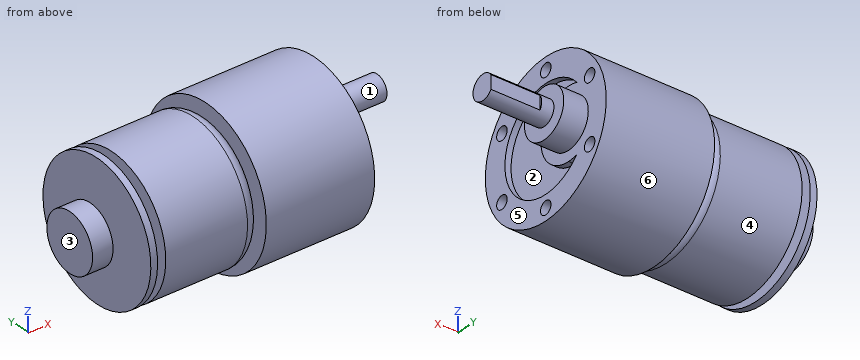
from build123d import *

# Parameters (mm, degrees)
CROQUIS_MOTOR_BASE_R      = 16.5
SALIENTE_EXTRUIR1_DEPTH   = 23
REDONDEO1_R               = 3
CROQUIS_REDUCTOR_BASE_R   = 18.5
SALIENTE_EXTRUIR2_DEPTH   = 26.5
CROQUIS_MOTOR_SHAFT_R     = 6
SALIENTE_EXTRUIR3_DEPTH   = 6
CORTAR_EXTRUIR1_DEPTH     = 1.5
CROQUIS_SHAFT_R           = 3
SALIENTE_EXTRUIR4_DEPTH   = 15
CORTAR_EXTRUIR2_START     = -12
CORTAR_EXTRUIR2_DEPTH     = 12
CROQUIS_MOUNT_AND_CLOSE_R = 1.6
CORTAR_EXTRUIR3_DEPTH     = 3
CROQUIS_MOTOR_SHAFT_OUT_R = 4
SALIENTE_EXTRUIR5_DEPTH   = 2
SALIENTE_EXTRUIR6_START   = 1.65
CROQUIS_ELECTRONICS_R     = 16.5
SALIENTE_EXTRUIR6_DEPTH   = 1.65
CROQUIS_MOTOR_AXIS_R      = 1
SALIENTE_EXTRUIR7_DEPTH   = 1.65
CROQUIS_ENCODER_R         = 7
SALIENTE_EXTRUIR8_DEPTH   = 5


with BuildPart() as part:
    # Croquis motor base → Saliente-Extruir1 (new body)
    with BuildSketch(Plane(origin=(0, 0, 0), x_dir=(0, 0, -1), z_dir=(1, 0, 0))):
        Circle(CROQUIS_MOTOR_BASE_R)
    extrude(amount=SALIENTE_EXTRUIR1_DEPTH)

    # Redondeo1
    redondeo1_edges = [part.edges().sort_by_distance(p)[0] for p in [
        (23, 0, 16.5),
    ]]
    fillet(redondeo1_edges, radius=REDONDEO1_R)

    # Croquis reductor base → Saliente-Extruir2 (add)
    with BuildSketch(Plane(origin=(23, 0, 0), x_dir=(0, 0, -1), z_dir=(1, 0, 0))):
        Circle(CROQUIS_REDUCTOR_BASE_R)
    extrude(amount=SALIENTE_EXTRUIR2_DEPTH)

    # Croquis motor shaft → Saliente-Extruir3 (add)
    with BuildSketch(Plane(origin=(49.5, 0, 0), x_dir=(0, 0, -1), z_dir=(1, 0, 0))):
        with Locations((0, 7)):
            Circle(CROQUIS_MOTOR_SHAFT_R)
    extrude(amount=SALIENTE_EXTRUIR3_DEPTH)

    # Croquis motor shaft_3 → Cortar-Extruir1 (cut)
    with BuildSketch(Plane(origin=(49.5, 0, 0), x_dir=(0, 0, -1), z_dir=(1, 0, 0))):
        with BuildLine():
            ThreePointArc((8.124038405, 9.5), (8.405484116, 8.264055687), (8.5, 7))
            ThreePointArc((8.5, 7), (-1.264055687, -1.405484116), (-8.124038405, 9.5))
            ThreePointArc((-8.124038405, 9.5), (0, -12.5), (8.124038405, 9.5))
        make_face()
    extrude(amount=-CORTAR_EXTRUIR1_DEPTH, mode=Mode.SUBTRACT)

    # Croquis shaft → Saliente-Extruir4 (add)
    with BuildSketch(Plane(origin=(55.5, 0, 0), x_dir=(0, 0, -1), z_dir=(1, 0, 0))):
        with Locations((0, 7)):
            Circle(CROQUIS_SHAFT_R)
    extrude(amount=SALIENTE_EXTRUIR4_DEPTH)

    # Croquis shaft lock → Cortar-Extruir2 (cut)
    with BuildSketch(Plane(origin=(70.5, 0, 0), x_dir=(0, 0, -1), z_dir=(1, 0, 0)).offset(CORTAR_EXTRUIR2_START)):
        with BuildLine():
            Line((-1.658312395, 9.5), (1.658312395, 9.5))
            ThreePointArc((1.658312395, 9.5), (0, 10), (-1.658312395, 9.5))
        make_face()
    extrude(amount=CORTAR_EXTRUIR2_DEPTH, mode=Mode.SUBTRACT)

    # Croquis mount and close → Cortar-Extruir3 (cut)
    with BuildSketch(Plane(origin=(49.5, 0, 0), x_dir=(0, 0, -1), z_dir=(1, 0, 0))):
        with Locations((-15.5, 0)):
            Circle(CROQUIS_MOUNT_AND_CLOSE_R)
        with Locations((-7.75, 13.423393759)):
            Circle(CROQUIS_MOUNT_AND_CLOSE_R)
        with Locations((7.75, 13.423393759)):
            Circle(CROQUIS_MOUNT_AND_CLOSE_R)
        with Locations((15.5, 0)):
            Circle(CROQUIS_MOUNT_AND_CLOSE_R)
        with Locations((7.75, -13.423393759)):
            Circle(CROQUIS_MOUNT_AND_CLOSE_R)
        with Locations((-7.75, -13.423393759)):
            Circle(CROQUIS_MOUNT_AND_CLOSE_R)
    extrude(amount=-CORTAR_EXTRUIR3_DEPTH, mode=Mode.SUBTRACT)

    # Croquis motor shaft out → Saliente-Extruir5 (add)
    with BuildSketch(Plane.ZY):
        Circle(CROQUIS_MOTOR_SHAFT_OUT_R)
    extrude(amount=SALIENTE_EXTRUIR5_DEPTH)

    # Croquis electronics → Saliente-Extruir6 (add)
    with BuildSketch(Plane.ZY.offset(2).offset(SALIENTE_EXTRUIR6_START)):
        with Locations(Location((0, 0, 0), (0, 0, 180))):
            Circle(CROQUIS_ELECTRONICS_R)
    extrude(amount=-SALIENTE_EXTRUIR6_DEPTH)

    # Croquis motor axis → Saliente-Extruir7 (add)
    with BuildSketch(Plane.ZY.offset(3.65)):
        Circle(CROQUIS_MOTOR_AXIS_R)
    extrude(amount=SALIENTE_EXTRUIR7_DEPTH)

    # Croquis encoder → Saliente-Extruir8 (add)
    with BuildSketch(Plane.ZY.offset(5.3)):
        Circle(CROQUIS_ENCODER_R)
    extrude(amount=SALIENTE_EXTRUIR8_DEPTH)


solid = part.part
Input: part model. Units: mm. Frame: model coordinates. Face numbers are marked on the shaded views. A direction names the side the tool comes from. Give positions to 0.01 mm unless a question says otherwise; leave off trailing zeros. Write each loop counter-clockwise with the first axis right and the second up, starting at its lowest first coordinate (ties: lowest second). Pieces come first, ordered by that corner, then holes. Notation, with made-up numbers: M 29,-13.75 L 81,-13.75 A24 cw 81,5.25 Z; hole C -38.5,67 d11. An arc over 180 degrees is marked long. Write item = value, one per line. Start each with the question number.
1) First-contact query: pin 1 Ø2 at (y, z) = (-1.5, -2) entering from +X; pin 2 Ø2.5 at (y, z) = (13.42, 7.75) entering from +X; pin 3 Ø8 at (x, z) = (25.5, -6.5) entering from +Y. Flat tips, straight axial feed; report the tip coordinate or a pass-through.
2) Draft query along Y for the marked faces 1, 2 and 3. Return one class per face: +Y half, -Y half, draft (parallel to the pull), parting line (faces both ways), or undercut.
3) Material intervals for line 1 along X through (y, z) = (-7, -8.5); line 2 along X through (y, z) = (-5, 11.5); line 3 along Y through (x, z) = (48.1, -7.75), sorted ascending. Write a range as [from, to].
4) Reachability of the marked faces 4, 5 and 6 from +Z, -Z, +X, -X, +Y, -Y: full face, straight path, thin tool, end or side. Return the list, or none.
5) Cut plane A-A on z = -15.5. Count the separate pieces of the cut face and the enclosed holes in it, then the cut area to 3 significant figures.
6) Cut plane B-B on x = 8. Return the cut outline in (y, z), then the cut area to 3 significant figures.
Solved:
q1.pin_1 = 49.5
q1.pin_2 = 46.5
q1.pin_3 = 18.33
q2.face_1 = parting line
q2.face_2 = undercut
q2.face_3 = draft
q3.line_1 = [-3.65, -2], [0, 48]
q3.line_2 = [-3.65, -2], [0, 49.5]
q3.line_3 = [-16.8, -15.02], [-11.82, -9.81], [3.51, 11.82], [15.02, 16.8]
q4.face_4 = -X
q4.face_5 = +X
q4.face_6 = +X, -X
q5.separate_pieces = 3
q5.enclosed_holes = 0
q5.area = 791 mm2
q6.outline = C 0,0 d33
q6.area = 855 mm2
